Could you check a few things on this model? Use its own coordinates, in mm. Coordinates: 2 decimals unless noted, no trailing zeros. Write each loop counter-clockwise with the first axis right and the second up, starting at its lowest first coordinate (ties: lowest second). Pieces come first, ordered by that corner, then holes. Notation, with made-up numbers: (3, 60.5) - (21, 60.5) arc R29 cw to (21, 82.5) - close; hole circle Ø9 at (49.5, 68.5). An arc over 180 degrees is marked (long way). Answer as a JSON object with one key per item and string values. Group by question number.
1) If we section it at B-B (z = 0): Write out the boundary of the cut face in (x, y).
2) We'd pull the mould along Z, two halves only. Please class faces 1 (the flat face through (0, 5, 0)), 2 (the flat face through (0.3, 0, -5.2)), 3 (the conical face through (4.81, 9.81, 21.66)), 4 (the cylindrical face through (4.88, 2.54, 1.08)): released by +Z, released by -Z, zero draft, split by the parting line, or undercut.
3) Will these pins go through, and if not, where does the flat tip stop? pin 1 Ø2 at (y, z) = (3.5, 6.5) entering from -X; pin 2 Ø3 at (x, y) = (2, 6) entering from +Z (3 decimals); pin 3 Ø3 at (y, z) = (7, -9.5) entering from -X.
4) If we section it at A-A (x = 0): Write out the boundary of the cut face in (y, z).
5) Please list where these lines run through material, in increasing order: line 1 along Z through (x, y) = (0, 1.85); line 2 along Z through (x, y) = (-17, 2.5); line 3 along X through (y, z) = (8.5, -11.5).
6) If we section it at C-C (y = 1.5): Write out the boundary of the cut face in (x, z).
Autodesk Inventor part; units mm, degrees
ref_plane "YZ Plane" through (0, 0, 0) normal (1, 0, 0) x (0, 1, 0)
ref_plane "XZ Plane" through (0, 0, 0) normal (0, 1, 0) x (-1, 0, 0)
ref_plane "XY Plane" through (0, 0, 0) normal (0, 0, 1) x (1, 0, 0)
sketch "Sketch1" plane through (0, 0, 0) normal (0, 1, 0) x (-1, 0, 0)
  circle A0 centre (0, 0) radius 25
  dimension "d0" = 50
extrude "Extrusion1" add sketch "Sketch1" along normal blind 10
chamfer "Chamfer1" distance 3 angle 45 1 edges at (25, 10, 0)
hole "Hole1" at (0, 0, 0) direction (0, 1, 0) diameter 10 depth 5
properties part number "stackLightTop" material "ABS Plastic"
Here are the results:
{
 "1": {"outline": "(-25, 0) - (-5, 0) - (-5, 5) - (5, 5) - (5, 0) - (25, 0) - (25, 7) - (22, 10) - (-22, 10) - (-25, 7) - close"},
 "2": {"face 1": "undercut", "face 2": "zero draft", "face 3": "split by the parting line", "face 4": "undercut"},
 "3": {"pin 1": "stops at x = -24.39", "pin 2": "stops at z = 24.995", "pin 3": "stops at x = -23.69"},
 "4": {"outline": "(0, -25) - (7, -25) - (10, -22) - (10, 22) - (7, 25) - (0, 25) - (0, 5) - (5, 5) - (5, -5) - (0, -5) - close"},
 "5": {"line 1": "z = -25 to -5, 5 to 25", "line 2": "z = -18.33 to 18.33", "line 3": "x = -20.49 to 20.49"},
 "6": {"outline": "circle Ø50 at (0, 0); hole circle Ø10 at (0, 0)"}
}
